The drawing under review shows one solid part. Ordinate dimensions are in mm from its lowest x, y, z. A direction names the side the tool comes from. Round coordinates to 2 decimals unless told otherwise and drop trailing zeros. Write each loop counter-clockwise with the first axis right and the second up, starting at its lowest first coordinate (ties: lowest second). Pieces come first, ordered by that corner, then holes. Notation, with made-up numbers: (-38, 67.5) - (-33, 67.5) arc R7 ccw to (-33, 73.5) - close; hole circle Ø3 at (0.25, 53). An arc over 180 degrees is marked (long way). Answer in a Markdown table with one row per item. Add a question column.
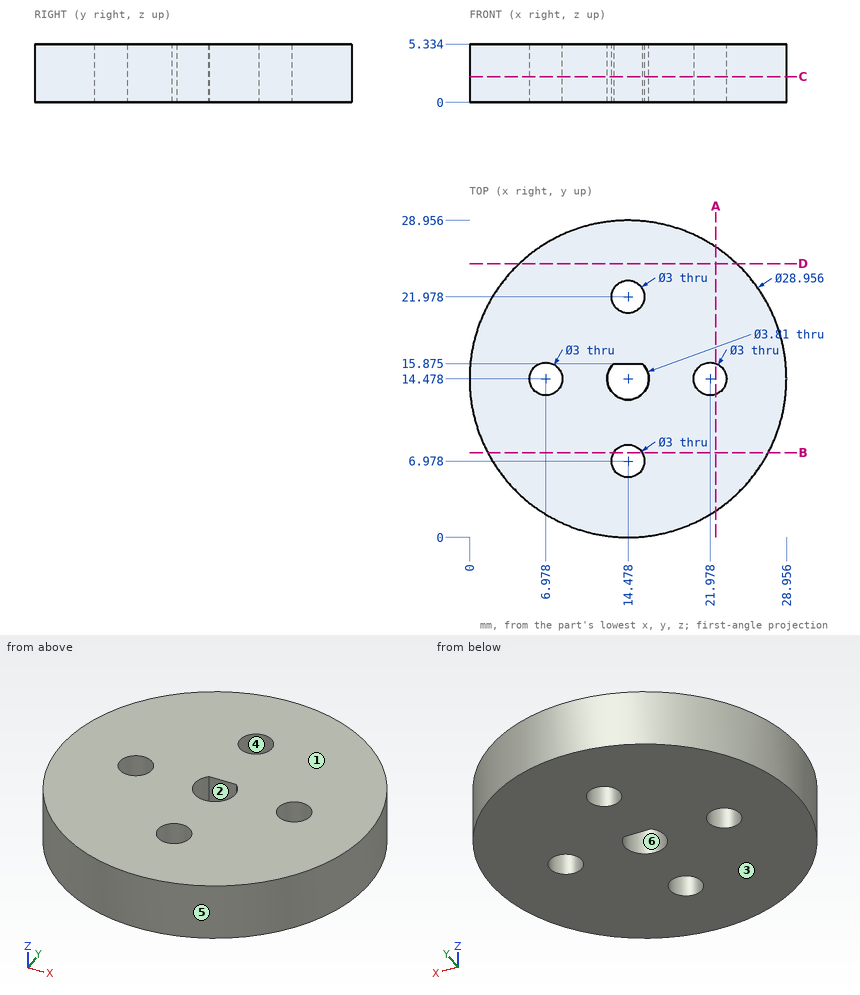
Q1. Add section B-B on y = 7.75. State the section outline as (x, z) points, then the cut area to 3 significant figures.
Q2. Draft analysis for pull direction X (two halves, no side actions). For the marked faces 3, 4, 5 and 6, state which applies: released by +X, released by -X, zero draft, split by the parting line, or undercut.
Q3. To check wall thickness, follow probe 1 along X at (y, z) = (14.25, 3.25); probe 2 along Y at (x, z) = (6.5, 2.1); probe 3 along Y at (x, z) = (15, 2.75) (3 decimals). State the ranges of each line that lie inside material, in increasing order.
Q4. Tool access review of the marked faces 1 and 2: name each direction out of +Z, -Z, +X, -X, +Y, -Y from which nothing blocks a thin tool from reaching the whole face with its end or side.
Q5. Add section C-C on z = 2.35. State the section outline as (x, y) points (3 decimals), then the cut area to 3 significant figures.
Q6. Insertion check: pin 1 Ø1.8 at (x, y) = (21.978, 14.478) entering from +Z; pin 2 Ø1.5 at (y, z) = (15.5, 1) entering from -X; pin 3 Ø1.5 at (x, z) = (22, 1) entering from -Y; pin 4 Ø2 at (y, z) = (18, 3) entering from -X. Each pin has a flat end and moves straight along its axis. Give the tip position at first contact, or say it passes through.
Q7. Add section D-D on y = 25. State the section outline as (x, z) points.
Q8. Add section A-A on x = 22.5. State the section outline as (y, z) points, then the cut area to 3 significant figures.
Answer sheet:
| question | item | result |
|---|---|---|
| 1 | outline | (1.66, 0) - (13.19, 0) - (13.19, 5.33) - (1.66, 5.33) - close; (15.76, 0) - (27.3, 0) - (27.3, 5.33) - (15.76, 5.33) - close |
| 1 | area | 123 mm² |
| 2 | face 3 | zero draft |
| 2 | face 4 | undercut |
| 2 | face 5 | split by the parting line |
| 2 | face 6 | undercut |
| 3 | probe 1 | x = 0 to 5.5, 8.46 to 12.59, 16.37 to 20.5, 23.46 to 28.95 |
| 3 | probe 2 | y = 2.4 to 13.06, 15.9 to 26.56 |
| 3 | probe 3 | y = 0.009 to 5.572, 8.384 to 12.646, 15.875 to 20.572, 23.384 to 28.947 |
| 4 | face 1 | +Z, +X, -X, +Y, -Y |
| 4 | face 2 | +Z, -Z |
| 5 | outline | circle Ø28.956 at (14.478, 14.478); hole circle Ø3 at (6.978, 14.478); hole circle Ø3 at (14.478, 6.978); hole circle Ø3 at (14.478, 21.978); hole (13.183, 15.875) arc R1.905 ccw (long way) to (15.773, 15.875) - close; hole circle Ø3 at (21.978, 14.478) |
| 5 | area | 620 mm² |
| 6 | pin 1 | passes through |
| 6 | pin 2 | stops at x = 0 |
| 6 | pin 3 | stops at y = 1.68 |
| 6 | pin 4 | stops at x = 0.22 |
| 7 | outline | (4.53, 0) - (24.42, 0) - (24.42, 5.33) - (4.53, 5.33) - close |
| 8 | outline | (2.43, 0) - (13.07, 0) - (13.07, 5.33) - (2.43, 5.33) - close; (15.88, 0) - (26.53, 0) - (26.53, 5.33) - (15.88, 5.33) - close |
| 8 | area | 114 mm² |
